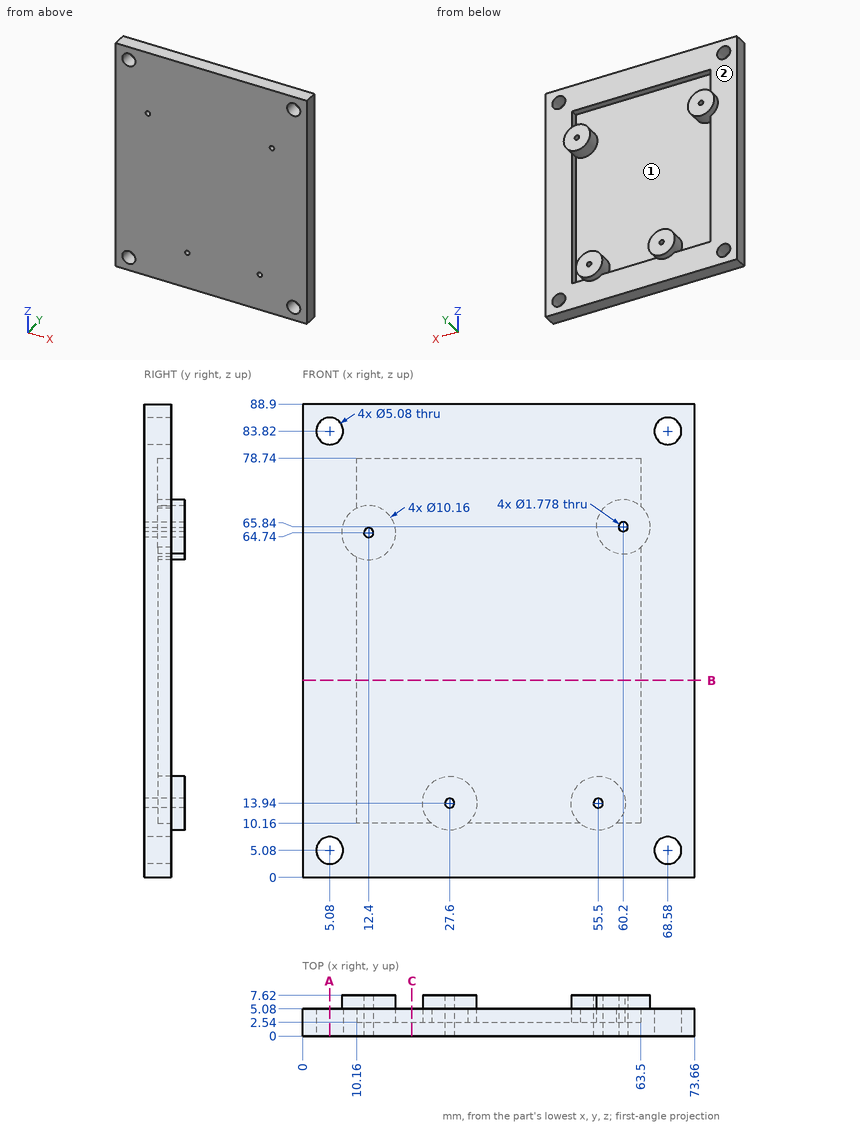
Geometry: see drawing. Coordinates: mm, zero at the bounding-box minimum. Coordinates: 2 decimals unless noted, no trailing zeros. Write each loop counter-clockwise with the first axis right and the second up, starting at its lowest first coordinate (ties: lowest second). Pieces come first, ordered by that corner, then holes.
1) Material intervals for line 1 along Z through (x, y) = (68.58, 2.25); line 2 along Z through (x, y) = (19, 4.5); line 3 along X through (y, z) = (2.75, 30), sorted ascending.
2) Pin query (flat end, axial travel): pin 1 Ø3 at (x, z) = (11, 74) entering from +Y; pin 2 Ø12 at (x, z) = (38, 40.5) entering from +Y; pin 3 Ø4.5 at (x, z) = (5.08, 5.08) entering from +Y. Return the tip coordinate at first contact, or that it passes through.
3) Mould query, pull axis Z, two halves, no side actions, for the marked faces 1 and 2. Classes: pulls with the +Z half, pulls with the -Z half, needs draft (parallel to the pull), parting line crosses it, or undercut.
4) Section A-A on x = 5.08. Output: boundary loops of the cut face in (y, z), and give its area (3 significant figures).
5) Section B-B on z = 37. Output: boundary loops of the cut face in (x, y).
6) Section C-C on x = 20.5. Output: boundary loops of the cut face in (y, z).
Check result:
1. line 1: z = 0 to 2.54, 7.62 to 81.28, 86.36 to 88.9
1. line 2: z = 0 to 10.16, 78.74 to 88.9
1. line 3: x = 0 to 10.16, 63.5 to 73.66
2. pin 1: stops at y = 5.08
2. pin 2: stops at y = 2.54
2. pin 3: passes through
3. face 1: undercut
3. face 2: needs draft
4. outline: (0, 0) - (5.08, 0) - (5.08, 2.54) - (0, 2.54) - close; (0, 7.62) - (5.08, 7.62) - (5.08, 81.28) - (0, 81.28) - close; (0, 86.36) - (5.08, 86.36) - (5.08, 88.9) - (0, 88.9) - close
4. area: 400 mm2
5. outline: (0, 0) - (73.66, 0) - (73.66, 5.08) - (63.5, 5.08) - (63.5, 2.54) - (10.16, 2.54) - (10.16, 5.08) - (0, 5.08) - close
6. outline: (0, 0) - (5.08, 0) - (5.08, 10.16) - (2.54, 10.16) - (2.54, 78.74) - (5.08, 78.74) - (5.08, 88.9) - (0, 88.9) - close
